from build123d import *

# Parameters (mm, degrees)
SKETCH1_R           = 2.7
SKETCH1_R_2         = 1.5
BOSS_EXTRUDE1_DEPTH = 5
SKETCH2_W           = 4.5
SKETCH2_H           = 5.9
BOSS_EXTRUDE2_DEPTH = 0.75
BOSS_EXTRUDE2_TAPER = 5


with BuildPart() as part:
    # Sketch1 → Boss-Extrude1 (new body)
    with BuildSketch(Plane.XY):
        with BuildLine():
            Line((0, -2), (0, -14))
            ThreePointArc((0, -14), (0.585786438, -15.414213562), (2, -16))
            Line((2, -16), (2.5, -16))
            ThreePointArc((2.5, -16), (3.914213562, -16.585786438), (4.5, -18))
            Line((4.5, -18), (4.5, -38))
            ThreePointArc((4.5, -38), (5.085786438, -39.414213562), (6.5, -40))
            Line((6.5, -40), (13, -40))
            ThreePointArc((13, -40), (14.414213562, -39.414213562), (15, -38))
            Line((15, -38), (15, -2))
            ThreePointArc((15, -2), (14.414213562, -0.585786438), (13, 0))
            Line((13, 0), (2, 0))
            ThreePointArc((2, 0), (0.585786438, -0.585786438), (0, -2))
        make_face()
        with Locations((7.5, -10)):
            Circle(SKETCH1_R, mode=Mode.SUBTRACT)
        with Locations((12, -34.8)):
            Circle(SKETCH1_R_2, mode=Mode.SUBTRACT)
        with Locations((12, -25.3)):
            Circle(SKETCH1_R_2, mode=Mode.SUBTRACT)
    extrude(amount=BOSS_EXTRUDE1_DEPTH)

    # Sketch2 → Boss-Extrude2 (add)
    with BuildSketch(Plane.XY.offset(5)):
        with Locations((2.25, -10)):
            Rectangle(SKETCH2_W, SKETCH2_H)
        with Locations((12.75, -10)):
            Rectangle(SKETCH2_W, SKETCH2_H)
    extrude(amount=BOSS_EXTRUDE2_DEPTH, taper=BOSS_EXTRUDE2_TAPER)


solid = part.part
Model file for the job. Use its own axes, mm. A direction names the side the tool comes from. Give positions to 0.01 mm unless a question says otherwise; leave off trailing zeros. Order: outer loops, then holes, each group sorted by start corner. A loop starts at its lowest first (then second) coordinate and runs counter-clockwise, first axis right, second up. Notation, with made-up numbers: (25, -10.5) - (38, -10.5) arc R17 ccw to (38, -3.5) - close; hole circle Ø8 at (-34.75, 86.25). An arc over 180 degrees is marked (long way). Return JSON: item names as keys, results as strings.
1) Cut at C-C, the plane x = 7.5. Give the cut face in (y, z), plus the area to 3 significant figures.
Geometry says:
{"outline": "(-40, 0) - (-12.7, 0) - (-12.7, 5) - (-40, 5) - close; (-7.3, 0) - (0, 0) - (0, 5) - (-7.3, 5) - close", "area": "173 mm²"}
2) Cut at A-A, the plane x = 12. Give the cut face in (y, z), plus the area to 3 significant figures.
Geometry says:
{"outline": "(-40, 0) - (-36.3, 0) - (-36.3, 5) - (-40, 5) - close; (-33.3, 0) - (-26.8, 0) - (-26.8, 5) - (-33.3, 5) - close; (-23.8, 0) - (0, 0) - (0, 5) - (-7.05, 5) - (-7.12, 5.75) - (-12.88, 5.75) - (-12.95, 5) - (-23.8, 5) - close", "area": "174 mm²"}
3) Cut at B-B, the plane y = -10. Give the cut face in (x, z), plus the area to 3 significant figures.
Geometry says:
{"outline": "(0, 0) - (4.8, 0) - (4.8, 5) - (4.5, 5) - (4.43, 5.75) - (0.07, 5.75) - (0, 5) - close; (10.2, 0) - (15, 0) - (15, 5) - (14.93, 5.75) - (10.57, 5.75) - (10.5, 5) - (10.2, 5) - close", "area": "54.7 mm²"}
4) Pull direction X, two halves, no side cores. Call faces 1 (the cylindrical face through (11.805, -23.813, 2.465)), 2 (the flat face through (13, -10, 5.75)), 3 (the cylindrical face through (9.994, -11.034, 2.465)), 4 (the cylindrical face through (5.07, -39.4, 2.46)): pulls with the +X half, pulls with the -X half, needs draft (parallel to the pull), parting line crosses it, or undercut.
Geometry says:
{"face 1": "undercut", "face 2": "needs draft", "face 3": "undercut", "face 4": "pulls with the -X half"}
5) 3-axis set-ups, long thin cutter, end or side, ignore diameter. For faces 5 (the flat face through (2, -10, 5.75)), 6 (the flat face through (4.5, -28, 2)): which of +Z, -Z, +X, -X, +Y, -Y reach the whole face in a straight line?
Geometry says:
{"face 5": "+Z, +X, -X, +Y, -Y", "face 6": "+Z, -Z, -X, -Y"}
6) Cut at D-D, the plane z = 1. Give the cut face in (x, y).
Geometry says:
{"outline": "(0, -14) arc R2 ccw to (2, -16) - (2.5, -16) arc R2 cw to (4.5, -18) - (4.5, -38) arc R2 ccw to (6.5, -40) - (13, -40) arc R2 ccw to (15, -38) - (15, -2) arc R2 ccw to (13, 0) - (2, 0) arc R2 ccw to (0, -2) - close; hole circle Ø5.4 at (7.5, -10); hole circle Ø3 at (12, -34.8); hole circle Ø3 at (12, -25.3)"}
7) Probe line 1 (Y direction, x = 12, z = 3.7); line 2 (Y direction, x = 7.5, z = 2.4); line 3 (Z direction, x = 8.25, y = -2). List the from-to ranges inside material, lowest first. Write a range as from..to.
Geometry says:
{"line 1": "-40..-36.3, -33.3..-26.8, -23.8..0", "line 2": "-40..-12.7, -7.3..0", "line 3": "0..5"}
8) Flat gauge pins, fed straight in: P1, Ø2.5, axis at x = 12, y = -25.3, coming from the -Z side; P2, Ø3.5, axis at x = 12, y = -34.8, coming from the +Z side; P3, Ø0.6, axis at x = 2, z = 2.5, coming from the -Y side; P4, Ø1.5, axis at x = 12, z = 3, coming from the +Y side. Where does each tip first touch, or does it go through?
Geometry says:
{"P1": "through", "P2": "z = 5", "P3": "y = -16", "P4": "y = 0"}
